The model under review builds one solid part; all positions refer to its coordinate system, in mm. Face numbers are marked on the shaded views. A direction names the side the tool comes from. Coordinates: 2 decimals unless noted, no trailing zeros. Write each loop counter-clockwise with the first axis right and the second up, starting at its lowest first coordinate (ties: lowest second). Pieces come first, ordered by that corner, then holes.
```python
from build123d import *

# Parameters (mm, degrees)
SKETCH_1_R               = 60
EXTRUDE_1_DEPTH          = 6
SKETCH_2_R               = 18
EXTRUDE_2_DEPTH          = 30
EXTRUDE_3_DEPTH          = 20
PATTERN_CIRCULAR_1_COUNT = 8
SKETCH_4_R               = 6
CUT_EXTRUDE_1_DEPTH      = 91
CHAMFER_1_SIZE           = 1


with BuildPart() as part:
    # Sketch 1 → Extrude 1 (new body)
    with BuildSketch(Plane.XY):
        Circle(SKETCH_1_R)
    extrude(amount=EXTRUDE_1_DEPTH)

    # Sketch 2 → Extrude 2 (add)
    with BuildSketch(Plane.XY):
        Circle(SKETCH_2_R)
    extrude(amount=EXTRUDE_2_DEPTH)

    # Sketch 3 → Extrude 3 (add)
    with BuildSketch(Plane.XY.offset(6)):
        with BuildLine():
            Line((10.793600627, 0.86952175), (11.31454516, -2.084901509))
            ThreePointArc((11.31454516, -2.084901509), (35.223702528, -5.567543346), (52.349392529, -22.611232566))
            Line((52.349392529, -22.611232566), (55.025968571, -21.256263675))
            ThreePointArc((55.025968571, -21.256263675), (36.565809219, -2.884494776), (10.793600627, 0.86952175))
        make_face()
    extrude_3 = extrude(amount=EXTRUDE_3_DEPTH)

    # Pattern Circular 1: Extrude 3 ×8 about axis
    pattern_circular_1_axis = Axis((0, 0, 0), (0, 0, 1))
    for i in range(1, PATTERN_CIRCULAR_1_COUNT):
        add(extrude_3.rotate(pattern_circular_1_axis, i * 360 / PATTERN_CIRCULAR_1_COUNT))

    # Sketch 4 → Cut-Extrude 1 (cut, through all)
    with BuildSketch(Plane.XY.offset(30)):
        Circle(SKETCH_4_R)
    extrude(amount=-CUT_EXTRUDE_1_DEPTH, mode=Mode.SUBTRACT)

    # Chamfer 1
    chamfer_1_edges = [part.edges().sort_by_distance(p)[0] for p in [
        (-18, 0, 30),
    ]]
    chamfer(chamfer_1_edges, length=CHAMFER_1_SIZE)


solid = part.part
```
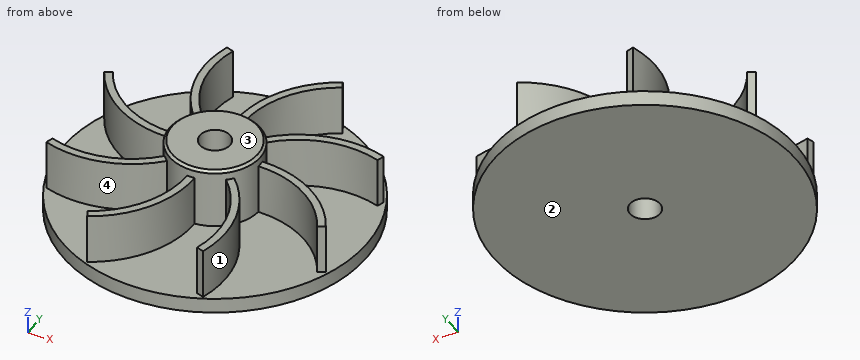
Item 1: Machinability: for the marked faces 3 and 4, which of the approach directions +Z, -Z, +X, -X, +Y, -Y give a long, thin tool a straight path to every point of the face, cutting with its end or side? Answer none if there is none.
Solved:
face 3: +Z, +X, -X, +Y, -Y
face 4: +Z
Item 2: Take a section at D-D, the plane x = -30. Write out the cut boundary in (y, z), plus the area to 3 significant figures.
Solved:
outline: (-51.96, 0) - (51.96, 0) - (51.96, 6) - (3.42, 6) - (3.42, 26) - (0.27, 26) - (0.27, 6) - (-21.34, 6) - (-21.34, 26) - (-24.46, 26) - (-24.46, 6) - (-51.96, 6) - close
area: 749 mm2
Item 3: Mouldability with a two-part tool opening along X and no side actions: class the marked faces 1 and 2 as pulls with the +X half, pulls with the -X half, needs draft (parallel to the pull), parting line crosses it, or undercut.
Solved:
face 1: undercut
face 2: needs draft
Item 4: For pin 1 (2 mm diameter, centred on y = 11, z = 24.5, fed in from -X); pin 2 (16 mm diameter, centred on x = 26.5, y = 21, fed in from +Z); pin 3 (4.5 mm diameter, centred on x = 17.5, y = -34.5, fed in from +Z), all flat-tipped, find the tip position at first contact; note any pin that passes through.
Solved:
pin 1: stops at x = -48.63
pin 2: stops at z = 26
pin 3: stops at z = 6
Item 5: To check wall thickness, follow line 1 along X through (y, z) = (16, 19.5); line 2 along X through (y, z) = (-18, 25.25). State the ranges of each line that lie inside material, in increasing order.
Solved:
line 1: x = -51.86 to -48.1, -17.56 to -13.71, -8.25 to 8.25, 14.06 to 18.96
line 2: x = -22.14 to -16.59, -1.5 to 1.5, 15.31 to 18.98, 49.6 to 53.19
Item 6: Take a section at A-A, the plane x = 0. Write out the cut boundary in (y, z).
Solved:
outline: (-60, 0) - (-6, 0) - (-6, 30) - (-17, 30) - (-18, 29) - (-18, 26) - (-29.06, 26) - (-29.06, 6) - (-60, 6) - close; (6, 0) - (60, 0) - (60, 6) - (29.06, 6) - (29.06, 26) - (18, 26) - (18, 29) - (17, 30) - (6, 30) - close
